```python
from build123d import *

# Parameters (mm, degrees)
SKETCH1_R            = 12.5
BOSS_EXTRUDE1_DEPTH  = 1.5
SKETCH2_R            = 40
SKETCH2_R_2          = 20
CUT_EXTRUDE1_DEPTH   = 0.5
FILLET1_R            = 10
FILLET1_OF_MIRROR1_R = 10


with BuildPart() as part:
    # Sketch1 → Boss-Extrude1 (new, symmetric)
    with BuildSketch(Plane.XY):
        with BuildLine():
            ThreePointArc((-4.982608643, 29.583333333), (-6.237350725, 29.344428022), (-7.480786198, 29.052329302))
            ThreePointArc((-7.480786198, 29.052329302), (-10.168416077, 22.838636441), (-16.584465184, 24.999110275))
            ThreePointArc((-16.584465184, 24.999110275), (-17.633557569, 24.270509831), (-18.650685145, 23.497913602))
            ThreePointArc((-18.650685145, 23.497913602), (-18.578620637, 16.728265159), (-25.31871703, 16.092313941))
            ThreePointArc((-25.31871703, 16.092313941), (-25.980762114, 15), (-26.595711193, 13.880495168))
            ThreePointArc((-26.595711193, 13.880495168), (-23.776412907, 7.725424859), (-29.675132687, 4.403010332))
            ThreePointArc((-29.675132687, 4.403010332), (-29.835656861, 3.135853898), (-29.942097162, 1.86301302))
            ThreePointArc((-29.942097162, 1.86301302), (-24.863047384, -2.613211582), (-28.900448313, -8.047613763))
            ThreePointArc((-28.900448313, -8.047613763), (-28.531695489, -9.270509831), (-28.111222517, -10.476601005))
            ThreePointArc((-28.111222517, -10.476601005), (-21.650635095, -12.5), (-23.128613874, -19.106732329))
            ThreePointArc((-23.128613874, -19.106732329), (-22.294344764, -20.073918191), (-21.419662115, -21.004715539))
            ThreePointArc((-21.419662115, -21.004715539), (-14.694631307, -20.225424859), (-13.357631979, -26.862123295))
            ThreePointArc((-13.357631979, -26.862123295), (-12.202099292, -27.406363729), (-11.024447543, -27.900923934))
            ThreePointArc((-11.024447543, -27.900923934), (-5.19779227, -24.453690018), (-1.276994164, -29.972809109))
            ThreePointArc((-1.276994164, -29.972809109), (0, -30), (1.276994164, -29.972809109))
            ThreePointArc((1.276994164, -29.972809109), (5.19779227, -24.453690018), (11.024447543, -27.900923934))
            ThreePointArc((11.024447543, -27.900923934), (12.202099292, -27.406363729), (13.357631979, -26.862123295))
            ThreePointArc((13.357631979, -26.862123295), (14.694631307, -20.225424859), (21.419662115, -21.004715539))
            ThreePointArc((21.419662115, -21.004715539), (22.294344764, -20.073918191), (23.128613874, -19.106732329))
            ThreePointArc((23.128613874, -19.106732329), (21.650635095, -12.5), (28.111222517, -10.476601005))
            ThreePointArc((28.111222517, -10.476601005), (28.531695489, -9.270509831), (28.900448313, -8.047613763))
            ThreePointArc((28.900448313, -8.047613763), (24.863047384, -2.613211582), (29.942097162, 1.86301302))
            ThreePointArc((29.942097162, 1.86301302), (29.835656861, 3.135853898), (29.675132687, 4.403010332))
            ThreePointArc((29.675132687, 4.403010332), (23.776412907, 7.725424859), (26.595711193, 13.880495168))
            ThreePointArc((26.595711193, 13.880495168), (25.980762114, 15), (25.31871703, 16.092313941))
            ThreePointArc((25.31871703, 16.092313941), (18.578620637, 16.728265159), (18.650685145, 23.497913602))
            ThreePointArc((18.650685145, 23.497913602), (17.633557569, 24.270509831), (16.584465184, 24.999110275))
            ThreePointArc((16.584465184, 24.999110275), (10.168416077, 22.838636441), (7.480786198, 29.052329302))
            ThreePointArc((7.480786198, 29.052329302), (6.237350725, 29.344428022), (4.982608643, 29.583333333))
            ThreePointArc((4.982608643, 29.583333333), (0, 25), (-4.982608643, 29.583333333))
        make_face()
        Circle(SKETCH1_R, mode=Mode.SUBTRACT)
    extrude(amount=BOSS_EXTRUDE1_DEPTH, both=True)

    # Sketch2 → Cut-Extrude1 (cut)
    with BuildSketch(Plane.XY.offset(1.5)):
        Circle(SKETCH2_R)
        Circle(SKETCH2_R_2, mode=Mode.SUBTRACT)
    cut_extrude1 = extrude(amount=-CUT_EXTRUDE1_DEPTH, mode=Mode.SUBTRACT)

    # Fillet1
    # the kernel refuses this fillet: 10 mm, written as the material it adds along each edge
    with BuildSketch(Plane(origin=(0, 0, 1), x_dir=(1, 0, 0), z_dir=(0, -1, 0))) as fillet1_piece_1:
        with BuildLine():
            CenterArc((23.122498999, 10), FILLET1_R, 251.805127661, 18.194872339)
            Line((20, 0.5), (19.93755002, 0.31))
            ThreePointArc((19.93755002, 0.31), (19.8, 0.25), (19.8, 0))
            Line((19.8, 0), (20, -0.2))
            Line((20, -0.2), (23.122498999, -0.2))
            Line((23.122498999, -0.2), (23.122498999, 0))
        make_face()
    revolve(axis=Axis((0, 0, 1), (0, 0, 1)))

    # Mirror1: Cut-Extrude1 across plane
    add(cut_extrude1.mirror(Plane.XY), mode=Mode.SUBTRACT)

    # Fillet1 of Mirror1
    # the kernel refuses this fillet: 10 mm, written as the material it adds along each edge
    with BuildSketch(Plane(origin=(0, 0, -1), x_dir=(1, 0, 0), z_dir=(0, -1, 0))) as fillet1_of_mirror1_piece_1:
        with BuildLine():
            CenterArc((23.122498999, -10), FILLET1_OF_MIRROR1_R, 90, 18.194872339)
            Line((20, -0.5), (19.93755002, -0.31))
            ThreePointArc((19.93755002, -0.31), (19.8, -0.25), (19.8, 0))
            Line((19.8, 0), (20, 0.2))
            Line((20, 0.2), (23.122498999, 0.2))
            Line((23.122498999, 0.2), (23.122498999, 0))
        make_face()
    revolve(axis=Axis((0, 0, -1), (0, 0, 1)))


solid = part.part
```
Build history of the part. All positions in model axes, mm. A direction names the side the tool comes from. Give positions to 0.01 mm unless a question says otherwise; leave off trailing zeros. Loops run counter-clockwise (first coordinate to the right, second up) from the corner with the lowest first, then second, coordinate; pieces in that order, holes last.
Item 1: Slice it at A-A, the plane x = 0. List the corners of the cut face in (y, z), and give its area (3 significant figures).
Answers follow:
outline: (-30, -1) - (-23.12, -1) arc R10 cw to (-20, -1.5) - (-12.5, -1.5) - (-12.5, 1.5) - (-20, 1.5) arc R10 cw to (-23.12, 1) - (-30, 1) - close; (12.5, -1.5) - (20, -1.5) arc R10 cw to (23.12, -1) - (25, -1) - (25, 1) - (23.12, 1) arc R10 cw to (20, 1.5) - (12.5, 1.5) - close
area: 77.1 mm2
Item 2: Slice it at D-D, the plane y = 0. List the corners of the cut face in (x, z), and give its area (3 significant figures).
Answers follow:
outline: (-25.94, -1) - (-23.12, -1) arc R10 cw to (-20, -1.5) - (-12.5, -1.5) - (-12.5, 1.5) - (-20, 1.5) arc R10 cw to (-23.12, 1) - (-25.94, 1) - close; (12.5, -1.5) - (20, -1.5) arc R10 cw to (23.12, -1) - (25.94, -1) - (25.94, 1) - (23.12, 1) arc R10 cw to (20, 1.5) - (12.5, 1.5) - close
area: 70.8 mm2
Item 3: Slice it at C-C, the plane y = 26. List the corners of the cut face in (x, z).
Answers follow:
outline: (-7.4, -1) - (-3, -1) - (-3, 1) - (-7.4, 1) - close; (3, -1) - (7.4, -1) - (7.4, 1) - (3, 1) - close
Item 4: Drill centre lines: line 1 (Y direction, x = 25.5, z = -0.35); line 2 (Z direction, x = 19, y = -14); line 3 (Y direction, x = 2.5, z = -0.6). Where is each one in solid material? Low to high.
Answers follow:
line 1: y = -10.02 to -5.63, -0.65 to 5.29, 13.25 to 15.8
line 2: z = -1 to 1
line 3: y = -26.02 to -12.25, 12.25 to 25.67
Item 5: Which spindle directions (+Z, -Z, +X, -X, +Y, -Y) get a long thin tool onto all of the face, cutting with end or side? Do faces 1 (the face through (21.6, -12.59, 0.01)), 2 (the face through (-16, 18, 1)). Say none if no direction does.
Answers follow:
face 1: +Z, -Z
face 2: +Z
Item 6: Flat gauge pins, fed straight in: pin 1 (1.5 mm diameter, centred on x = 17, y = -16, fed in from +Z); pin 2 (6 mm diameter, centred on x = -6, y = -24, fed in from -Z); pin 3 (2 mm diameter, centred on x = 12, y = 21, fed in from -Z). Where does each tip first touch, or does it go through?
Answers follow:
pin 1: stops at z = 1.01
pin 2: stops at z = -1.1
pin 3: stops at z = -1
Item 7: Pull direction Y, two halves, no side cores. Call faces 3 (the face through (14.61, -20.29, 0.01)), 4 (the face through (29.838, 3.118, 0.014)), 5 (the face through (-22.306, -20.061, 0.014)): released by +Y, released by -Y, zero draft, split by the parting line, or undercut.
Answers follow:
face 3: undercut
face 4: released by +Y
face 5: released by -Y
